Geometry: see drawing. Coordinates: mm, zero at the bounding-box minimum. A direction names the side the tool comes from. Give positions to 0.01 mm unless a question says otherwise; leave off trailing zeros. Write each loop counter-clockwise with the first axis right and the second up, starting at its lowest first coordinate (ties: lowest second). Pieces come first, ordered by that corner, then holes. Notation, with made-up numbers: (-8, 46.5) - (38, 46.5) arc R33 cw to (38, 74.5) - close; hole circle Ø3 at (45, 56). An arc over 180 degrees is marked (long way). Use CSV: the item, a comma, the result in double quotes. Start each with the question number.
(1) Section D-D on z = 4.75. Output: boundary loops of the cut face in (x, y) (1 decimal).
(2) Line query: probe 1 along Y at (x, z) = (25, 28); probe 2 along X at (y, z) = (7, 21); probe 3 along Y at (x, z) = (6, 21.75). Output: solid intervals per line, ascending. Write a range as [from, to].
(3) Section C-C on y = 36. Output: boundary loops of the cut face in (x, z).
(4) Draft query along Z for the marked faces 1, 2, 3 and 4. Return one class per face: released by +Z, released by -Z, zero draft, split by the parting line, or undercut.
(5) Section B-B on x = 23. Output: boundary loops of the cut face in (y, z), and give its area (3 significant figures).
(6) Reachability of the marked faces 5, 6 and 7 from +Z, -Z, +X, -X, +Y, -Y: full face, straight path, thin tool, end or side. Return the list, or none.
(7) First-contact query: pin 1 Ø1.5 at (x, z) = (32, 23) entering from +Y; pin 2 Ø10 at (x, y) = (44, 28.5) entering from -Z; pin 3 Ø4 at (y, z) = (7, 20.5) entering from -X; pin 4 Ø4 at (x, z) = (3.5, 14) entering from -Y. Flat tips, straight axial feed; report the tip coordinate or a pass-through.
(8) Section A-A on z = 15. Output: boundary loops of the cut face in (x, y) (1 decimal).
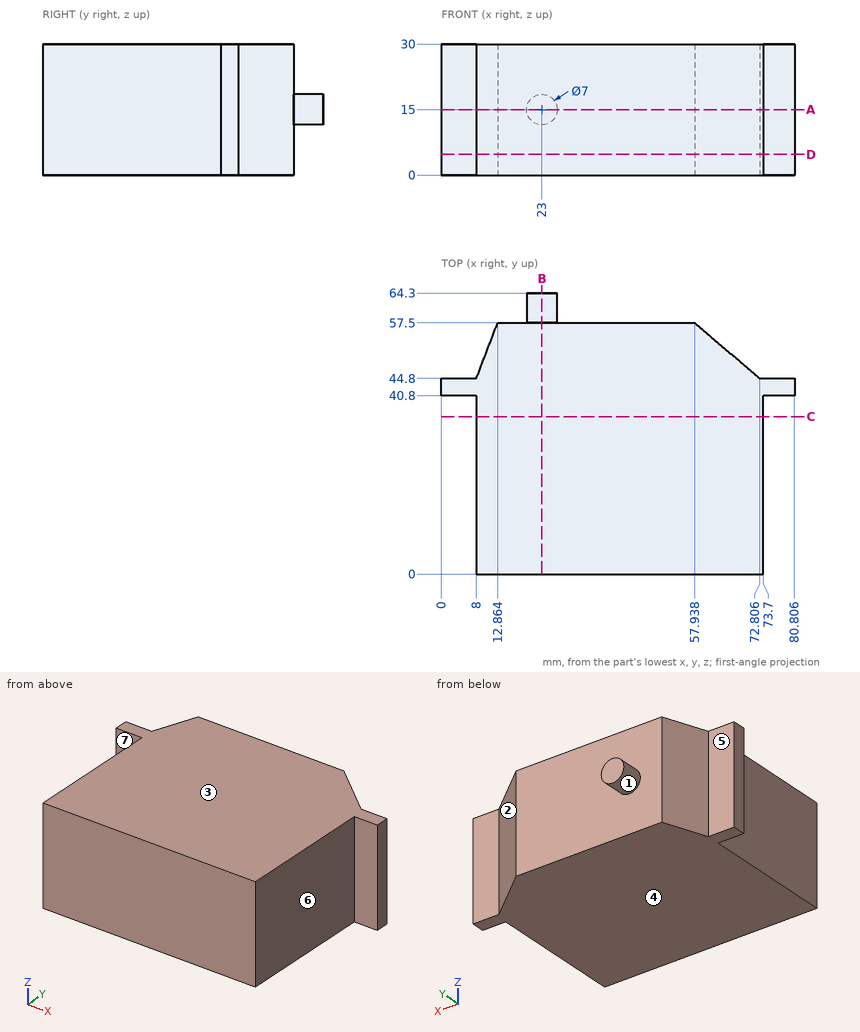
Check values:
1,outline,"(0, 40.8) - (8, 40.8) - (8, 0) - (73.7, 0) - (73.7, 40.8) - (80.8, 40.8) - (80.8, 44.8) - (72.8, 44.8) - (57.9, 57.5) - (12.9, 57.5) - (8, 44.8) - (0, 44.8) - close"
2,probe 1,"y = [0, 57.5]"
2,probe 2,"x = [8, 73.7]"
2,probe 3,"y = [40.8, 44.8]"
3,outline,"(8, 0) - (73.7, 0) - (73.7, 30) - (8, 30) - close"
4,face 1,"split by the parting line"
4,face 2,"zero draft"
4,face 3,"released by +Z"
4,face 4,"released by -Z"
5,outline,"(0, 0) - (57.5, 0) - (57.5, 11.5) - (64.3, 11.5) - (64.3, 18.5) - (57.5, 18.5) - (57.5, 30) - (0, 30) - close"
5,area,"1,770 mm²"
6,face 5,"+Z, -Z, -X, +Y"
6,face 6,"+Z, -Z, +X, -Y"
6,face 7,"+Z, -Z, -X, -Y"
7,pin 1,"stops at y = 57.5"
7,pin 2,"stops at z = 0"
7,pin 3,"stops at x = 8"
7,pin 4,"stops at y = 40.8"
8,outline,"(0, 40.8) - (8, 40.8) - (8, 0) - (73.7, 0) - (73.7, 40.8) - (80.8, 40.8) - (80.8, 44.8) - (72.8, 44.8) - (57.9, 57.5) - (26.5, 57.5) - (26.5, 64.3) - (19.5, 64.3) - (19.5, 57.5) - (12.9, 57.5) - (8, 44.8) - (0, 44.8) - close"
